Verification items for the finished model (mm, model axes). A direction names the side the tool comes from. Round coordinates to 2 decimals unless told otherwise and drop trailing zeros. Write each loop counter-clockwise with the first axis right and the second up, starting at its lowest first coordinate (ties: lowest second). Pieces come first, ordered by that corner, then holes. Notation, with made-up numbers: (80.25, 63.5) - (119.25, 63.5) arc R20 cw to (119.25, 73.5) - close; hole circle Ø2 at (76, 71). An arc over 180 degrees is marked (long way). Write each question's results on one line, items separated by ' | '.
```python
from build123d import *

# Parameters (mm, degrees)
ESQUISSE1_W             = 15
ESQUISSE1_H             = 83
BOSS_EXTRU_1_DEPTH      = 6
ESQUISSE2_R             = 11
BOSS_EXTRU_2_DEPTH      = 6
ESQUISSE4_R             = 4
ESQUISSE4_R_2           = 1.005
ESQUISSE4_R_3           = 6.45
ENL_V_MAT_EXTRU_2_DEPTH = 10
ESQUISSE5_R             = 2
ENL_V_MAT_EXTRU_3_DEPTH = 4


with BuildPart() as part:
    # Esquisse1 → Boss.-Extru.1 (new body)
    with BuildSketch(Plane.XY):
        with Locations((7.5, 41.5)):
            Rectangle(ESQUISSE1_W, ESQUISSE1_H)
    extrude(amount=BOSS_EXTRU_1_DEPTH)

    # Esquisse2 → Boss.-Extru.2 (add)
    with BuildSketch(Plane.XY.offset(6)):
        with Locations((7.5, 7.5)):
            Circle(ESQUISSE2_R)
        with Locations((7.5, 75.5)):
            Circle(ESQUISSE2_R)
    extrude(amount=-BOSS_EXTRU_2_DEPTH)

    # Esquisse4 → Enlèv. mat.-Extru.2 (cut)
    with BuildSketch(Plane(origin=(0, 0, 0), x_dir=(-1, 0, 0), z_dir=(0, 0, -1))):
        with Locations((-7.5, 75.5)):
            Circle(ESQUISSE4_R)
        with Locations((-7.5, 67.5)):
            Circle(ESQUISSE4_R_2)
        with Locations((-15.5, 75.5)):
            Circle(ESQUISSE4_R_2)
        with Locations((-7.5, 83.5)):
            Circle(ESQUISSE4_R_2)
        with Locations((0.5, 75.5)):
            Circle(ESQUISSE4_R_2)
        with Locations((-7.5, 7.5)):
            Circle(ESQUISSE4_R_3)
    extrude(amount=-ENL_V_MAT_EXTRU_2_DEPTH, mode=Mode.SUBTRACT)

    # Esquisse5 → Enlèv. mat.-Extru.3 (cut)
    with BuildSketch(Plane(origin=(0, 0, 0), x_dir=(-1, 0, 0), z_dir=(0, 0, -1))):
        with Locations((-15.5, 75.5)):
            Circle(ESQUISSE5_R)
        with Locations((-7.5, 83.5)):
            Circle(ESQUISSE5_R)
        with Locations((0.5, 75.5)):
            Circle(ESQUISSE5_R)
        with Locations((-7.5, 67.5)):
            Circle(ESQUISSE5_R)
    extrude(amount=-ENL_V_MAT_EXTRU_3_DEPTH, mode=Mode.SUBTRACT)


solid = part.part
```
(1) Section check D-D (x = 12.5). Record the cut outline in (y, z), plus the area to 3 significant figures.
Answer:
outline: (-2.3, 0) - (3.43, 0) - (3.43, 6) - (-2.3, 6) - close; (11.57, 0) - (85.3, 0) - (85.3, 6) - (11.57, 6) - close | area: 477 mm2
(2) Thickness scan on L1, parallel to Y at x = 7.5, z = 2.5; L2, parallel to Y at x = 7.5, z = 5.4 (3 decimals); L3, parallel to Y at x = 5, z = 5.2. Record the ranges inside material, lowest first.
Answer:
L1: -3.5 to 1.05, 13.95 to 65.5, 69.5 to 71.5, 79.5 to 81.5, 85.5 to 86.5 | L2: -3.5 to 1.05, 13.95 to 66.495, 68.505 to 71.5, 79.5 to 82.495, 84.505 to 86.5 | L3: -3.21 to 1.55, 13.45 to 72.38, 78.62 to 86.21
(3) Set-up check for faces 1 (the cylindrical face through (-0.24, 77.483, 1.972)), 2 (the flat face through (15, 41, 3)), 3 (the cylindrical face through (8.367, 71.595, 2.958)): record each of +Z, -Z, +X, -X, +Y, -Y from which the full face is reachable in a straight line by a thin tool's end or side.
Answer:
face 1: -Z | face 2: +Z, -Z, +X | face 3: +Z, -Z
(4) Section check C-C (y = 7.5). Record the cut outline in (x, z), plus the area to 3 significant figures.
Answer:
outline: (-3.5, 0) - (1.05, 0) - (1.05, 6) - (-3.5, 6) - close; (13.95, 0) - (18.5, 0) - (18.5, 6) - (13.95, 6) - close | area: 54.6 mm2
(5) Mould release check, pull along X, two halves, no side actions. Record for faces 4 (the flat face through (6.6, 82.6, 4)), 5 (the flat face through (0, 41, 3)), 6 (the cylindrical face through (7.132, -3.494, 3.042)): released by +X, released by -X, zero draft, split by the parting line, or undercut.
Answer:
face 4: undercut | face 5: released by -X | face 6: split by the parting line
(6) Section check B-B (x = 7.5). Record the cut outline in (y, z) (3 decimals), plus the area to 3 significant figures.
Answer:
outline: (-3.5, 0) - (1.05, 0) - (1.05, 6) - (-3.5, 6) - close; (13.95, 0) - (65.5, 0) - (65.5, 4) - (66.495, 4) - (66.495, 6) - (13.95, 6) - close; (68.505, 4) - (69.5, 4) - (69.5, 0) - (71.5, 0) - (71.5, 6) - (68.505, 6) - close; (79.5, 0) - (81.5, 0) - (81.5, 4) - (82.495, 4) - (82.495, 6) - (79.5, 6) - close; (84.505, 4) - (85.5, 4) - (85.5, 0) - (86.5, 0) - (86.5, 6) - (84.505, 6) - close | area: 375 mm2
(7) Go/stop test with flat-tipped pins: pin 1 Ø1 at (x, z) = (4, 3.5) entering from -Y; pin 2 Ø2 at (x, y) = (15.5, 76) entering from -Z; pin 3 Ø1 at (y, z) = (10.5, 2) entering from -X; pin 4 Ø1.8 at (x, y) = (7.5, 67.5) entering from +Z. Record where each tip stops, or that it passes through.
Answer:
pin 1: y = -3.08 | pin 2: z = 4 | pin 3: x = -3.21 | pin 4: through
(8) Section check A-A (z = 5.2). Record the cut outline in (x, y) (3 decimals).
Answer:
outline: (0, 15.547) arc R11 ccw (long way) to (15, 15.547) - (15, 67.453) arc R11 ccw (long way) to (0, 67.453) - close; hole circle Ø2.01 at (-0.5, 75.5); hole circle Ø12.9 at (7.5, 7.5); hole circle Ø8 at (7.5, 75.5); hole circle Ø2.01 at (7.5, 67.5); hole circle Ø2.01 at (7.5, 83.5); hole circle Ø2.01 at (15.5, 75.5)
